Check sheet for the drawn part. Datum: minimum x, y, z corner. Units: mm. A direction names the side the tool comes from. Give positions to 0.01 mm unless a question says otherwise; leave off trailing zeros. Loops run counter-clockwise (first coordinate to the right, second up) from the corner with the lowest first, then second, coordinate; pieces in that order, holes last. Notation, with made-up numbers: M 61,22.25 L 70,22.25 A20 ccw 70,28.25 Z; hole C -13,16.25 d1. An arc over 180 degrees is marked long. Write each question's results on one line, items separated by ' | '. Start each with the question number.
1. Sectioned sample at B-B on y = 54.5. Record the cut outline in (x, z).
2. Sectioned sample at A-A on z = 157. Record the cut outline in (x, y), and give its area (3 significant figures).
3. Sectioned sample at C-C on x = 33. Record the cut outline in (y, z).
4. Draft check along Z on the marked faces 6, 7 and 8. Enter one of: pulls with the +Z half, pulls with the -Z half, needs draft (parallel to the pull), parting line crosses it, or undercut.
5. Material ranges on line 1 along X through (y, z) = (58.5, 180); line 2 along Z through (x, y) = (46, 163.5); line 3 along Z through (x, y) = (67.5, 41.5), recorded low to high.
6. Tool access check on the marked faces 1, 2, 3, 4 and 5. Record the directions out of +Z, -Z, +X, -X, +Y, -Y that give a thin tool (end or side, any length) a straight path to the whole face; none if there is none.
7. Sectioned sample at D-D on z = 27.5. Record the cut outline in (x, y).
8. Go/stop test with flat-tipped pins: pin 1 (20.5 mm diameter, centred on y = 48.5, z = 189.5, fed in from -X); pin 2 (20.5 mm diameter, centred on x = 98.5, z = 175.5, fed in from -Y); pin 3 (15 mm diameter, centred on y = 35.5, z = 158, fed in from +X). Record where each tip stops, or that it passes through.
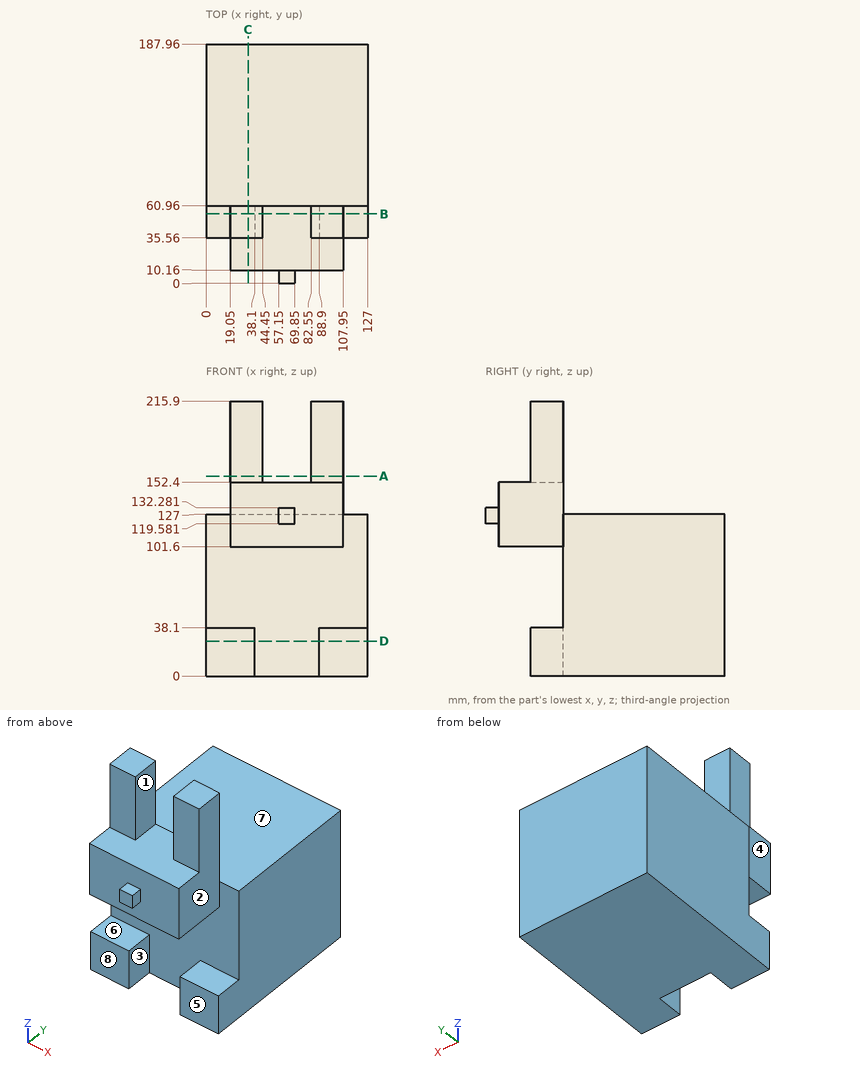
Output values:
1) outline: M 0,0 L 38.1,0 L 38.1,38.1 L 0,38.1 Z; M 19.05,101.6 L 107.95,101.6 L 107.95,215.9 L 82.55,215.9 L 82.55,152.4 L 44.45,152.4 L 44.45,215.9 L 19.05,215.9 Z; M 88.9,0 L 127,0 L 127,38.1 L 88.9,38.1 Z
2) outline: M 19.05,35.56 L 44.45,35.56 L 44.45,60.96 L 19.05,60.96 Z; M 82.55,35.56 L 107.95,35.56 L 107.95,60.96 L 82.55,60.96 Z | area: 1,290 mm2
3) outline: M 10.16,101.6 L 60.96,101.6 L 60.96,38.1 L 35.56,38.1 L 35.56,0 L 187.96,0 L 187.96,127 L 60.96,127 L 60.96,215.9 L 35.56,215.9 L 35.56,152.4 L 10.16,152.4 Z
4) face 6: undercut | face 7: pulls with the +Z half | face 8: needs draft
5) line 1: 19.05 to 44.45, 82.55 to 107.95 | line 2: 0 to 127 | line 3: 101.6 to 152.4
6) face 1: +Z, +Y, -Y | face 2: +Z, +X, -Y | face 3: -Z, -Y | face 4: +Z, -X, -Y | face 5: -Z, +X, -X, -Y
7) outline: M 0,35.56 L 38.1,35.56 L 38.1,60.96 L 88.9,60.96 L 88.9,35.56 L 127,35.56 L 127,187.96 L 0,187.96 Z
8) pin 1: x = 19.05 | pin 2: y = 35.56 | pin 3: x = 107.95
